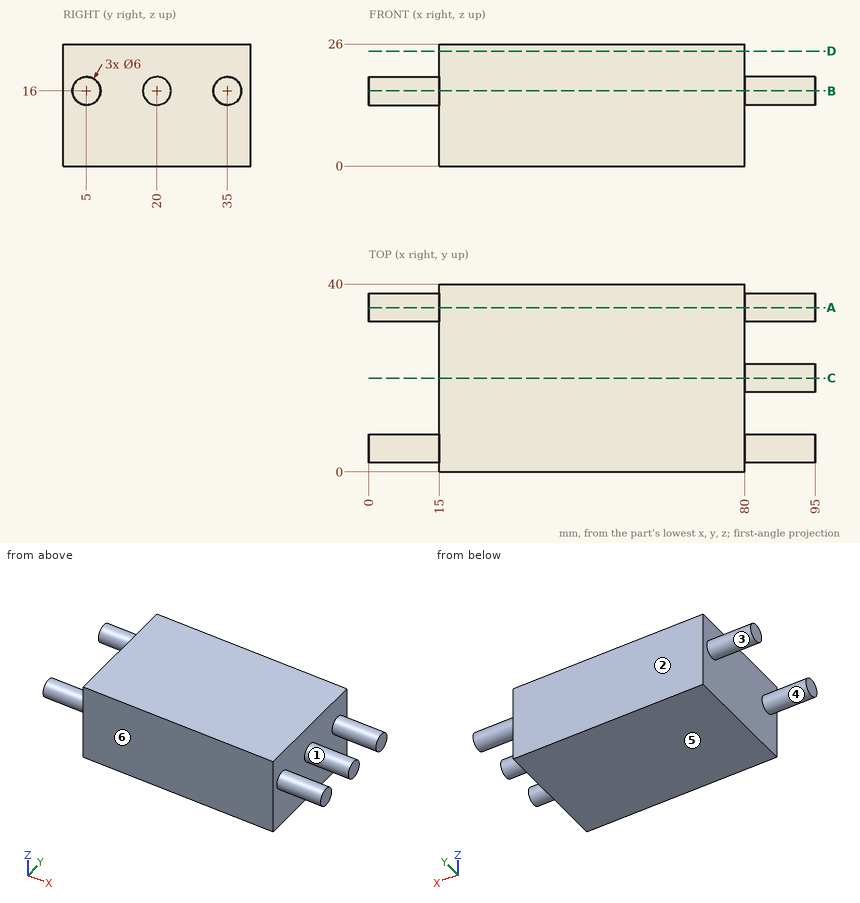
Input: dimensioned drawing with shaded views. Units: mm. Origin: part minimum x, y, z. A direction names the side the tool comes from. Coordinates: 2 decimals unless noted, no trailing zeros. Write each loop counter-clockwise with the first axis right and the second up, starting at its lowest first coordinate (ties: lowest second). Pieces come first, ordered by that corner, then holes. Notation, with made-up numbers: M 66,10.25 L 94,10.25 A33 ccw 94,40.25 Z; hole C -38.75,-31.75 d7. An arc over 180 degrees is marked long. Answer as CSV lines item,"result". Start each with the question number.
Q1. Reachability of the marked faces 1, 2 and 3 from +Z, -Z, +X, -X, +Y, -Y: full face, straight path, thin tool, end or side. Return the list, or none.
Q2. Pin query (flat end, axial travel): P1, Ø1.5, axis at x = 12.5, y = 6.5, coming from the -Z side; P2, Ø5, axis at y = 30, z = 7, coming from the +X side; P3, Ø4, axis at y = 28, z = 19.5, coming from the -X side. Return the tip coordinate at first contact, or that it passes through.
Q3. Cut plane D-D on z = 24.5. Return the cut outline in (x, y), then the cut area to 3 significant figures.
Q4. Cut plane C-C on y = 20. Return the cut outline in (x, z), then the cut area to 3 significant figures.
Q5. Cut plane A-A on y = 35. Return the cut outline in (x, z), then the cut area to 3 significant figures.
Q6. Cut plane B-B on z = 16. Return the cut outline in (x, y).
Q7. Mould query, pull axis Y, two halves, no side actions, for the marked faces 4, 5 and 6. Classes: released by +Y, released by -Y, zero draft, split by the parting line, or undercut.
Q8. Line query: line 1 (Y direction, x = 89.5, z = 18); line 2 (X direction, y = 35.5, z = 2.25); line 3 (Y direction, x = 5.5, z = 17.75). Output: solid intervals per line, ascending. Write a range as from..to.
Findings below:
1,face 1,"+X"
1,face 2,"+Z, -Z, +X, -X, +Y"
1,face 3,"-X"
2,P1,"stops at z = 13.1"
2,P2,"stops at x = 80"
2,P3,"stops at x = 15"
3,outline,"M 15,0 L 80,0 L 80,40 L 15,40 Z"
3,area,"2,600 mm2"
4,outline,"M 15,0 L 80,0 L 80,13 L 95,13 L 95,19 L 80,19 L 80,26 L 15,26 Z"
4,area,"1,780 mm2"
5,outline,"M 0,13 L 15,13 L 15,0 L 80,0 L 80,13 L 95,13 L 95,19 L 80,19 L 80,26 L 15,26 L 15,19 L 0,19 Z"
5,area,"1,870 mm2"
6,outline,"M 0,2 L 15,2 L 15,0 L 80,0 L 80,2 L 95,2 L 95,8 L 80,8 L 80,17 L 95,17 L 95,23 L 80,23 L 80,32 L 95,32 L 95,38 L 80,38 L 80,40 L 15,40 L 15,38 L 0,38 L 0,32 L 15,32 L 15,8 L 0,8 Z"
7,face 4,"undercut"
7,face 5,"zero draft"
7,face 6,"released by -Y"
8,line 1,"y = 2.76..7.24, 17.76..22.24, 32.76..37.24"
8,line 2,"x = 15..80"
8,line 3,"y = 2.56..7.44, 32.56..37.44"
